Work out the finished part from the listing and answer in its coordinate system (mm). Face numbers are marked on the shaded views. A direction names the side the tool comes from. Coordinates: 2 decimals unless noted, no trailing zeros. Order: outer loops, then holes, each group sorted by start corner. A loop starts at its lowest first (then second) coordinate and runs counter-clockwise, first axis right, second up. Notation, with made-up numbers: (12, 89) - (38, 89) arc R21 ccw to (38, 127) - close; hole circle Ø6 at (7, -29.75). An arc over 180 degrees is marked (long way). Answer as a JSON object with one key per item and string values. Group by question number.
1) Section A-A (x = -41.5) is taken. Give the vertices of the cut face in (y, z).
2) Each of these flat-tipped pins is pushed along its axis until it touches: P1, Ø20, axis at y = -1.5, z = 14, coming from the -X side; P2, Ø9, axis at y = -8, z = 20, coming from the +X side. Where does it stop, or does it pass through?
3) Section C-C (y = 26) is taken. Give the vertices of the cut face in (x, z), plus the area to 3 significant figures.
4) Find the intervals of material crossed by line 1 along Y through (x, z) = (-31.85, 20); line 2 along Y through (x, z) = (-46, 34); line 3 along X through (y, z) = (-15, 4), in increasing order.
5) Section D-D (z = 27) is taken. Give the vertices of the cut face in (x, y).
6) Section B-B (z = 10) is taken. Give the vertices of the cut face in (x, y).
7) A tool of negligible diameter and unlimited length cuts with its end or side. For the marked faces 1 and 2, from which of +Z, -Z, +X, -X, +Y, -Y can it reach the whole face along a straight path? Write none if from no direction.
8) The mould has two halves that part along Y. Classify the marked faces 3, 4 and 5: released by +Y, released by -Y, zero draft, split by the parting line, or undercut.
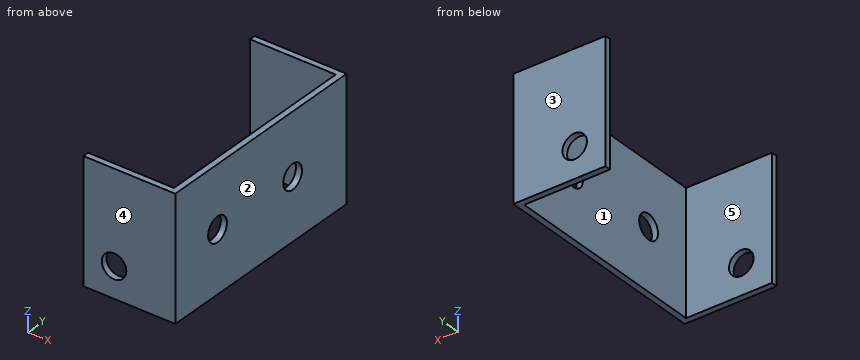
from build123d import *

# Parameters (mm, degrees)
EXTRUDE_1_DEPTH     = 40
SKETCH_3_R          = 4
CUT_EXTRUDE_1_DEPTH = 40
SKETCH_4_R          = 4
CUT_EXTRUDE_2_DEPTH = 96


with BuildPart() as part:
    # 草图1 → 凸台-拉伸1 (new body)
    with BuildSketch(Plane.XY):
        Polygon((-61.165760894, 46.995024588), (-31.165760894, 46.995024588), (-31.165760894, -26.004975412), (-61.165760894, -26.004975412), (-61.165760894, -24.004975412), (-33.165760894, -24.004975412), (-33.165760894, 44.995024588), (-61.165760894, 44.995024588), align=None)
    extrude(amount=EXTRUDE_1_DEPTH)

    # 草图3 → 切除-拉伸1 (cut)
    with BuildSketch(Plane.ZY.offset(33.165760894)):
        with Locations((20, 23.995024588)):
            Circle(SKETCH_3_R)
        with Locations((20, -8.004975412)):
            Circle(SKETCH_3_R)
    extrude(amount=-CUT_EXTRUDE_1_DEPTH, mode=Mode.SUBTRACT)

    # 草图4 → 切除-拉伸2 (cut)
    with BuildSketch(Plane(origin=(0, 46.995024588, 0), x_dir=(1, 0, 0), z_dir=(0, 1, 0))):
        with Locations((-51.165760894, -10)):
            Circle(SKETCH_4_R)
    extrude(amount=-CUT_EXTRUDE_2_DEPTH, mode=Mode.SUBTRACT)


solid = part.part
Report:
{
 "1": {"outline": "(-26, 0) - (-24, 0) - (-24, 40) - (-26, 40) - close; (45, 0) - (47, 0) - (47, 40) - (45, 40) - close"},
 "2": {"P1": "stops at x = -33.17", "P2": "stops at x = -31.17"},
 "3": {"outline": "(-33.17, 0) - (-31.17, 0) - (-31.17, 16.54) - (-33.17, 16.54) - close; (-33.17, 23.46) - (-31.17, 23.46) - (-31.17, 40) - (-33.17, 40) - close", "area": "66.2 mm²"},
 "4": {"line 1": "y = -26 to -12, -4 to 20, 28 to 47", "line 2": "y = -26 to -24, 45 to 47", "line 3": "x = -33.17 to -31.17"},
 "5": {"outline": "(-61.17, -26) - (-31.17, -26) - (-31.17, 47) - (-61.17, 47) - (-61.17, 45) - (-33.17, 45) - (-33.17, -24) - (-61.17, -24) - close"},
 "6": {"outline": "(-61.17, -26) - (-55.17, -26) - (-55.17, -24) - (-61.17, -24) - close; (-61.17, 45) - (-55.17, 45) - (-55.17, 47) - (-61.17, 47) - close; (-47.17, -26) - (-31.17, -26) - (-31.17, 47) - (-47.17, 47) - (-47.17, 45) - (-33.17, 45) - (-33.17, -24) - (-47.17, -24) - close"},
 "7": {"face 1": "+Z, -Z, -X", "face 2": "+Z, -Z, +X, +Y, -Y"},
 "8": {"face 3": "released by +Y", "face 4": "released by -Y", "face 5": "undercut"}
}
